```python
from build123d import *

# Parameters (mm, degrees)
F0_W     = 2
F0_H     = 0.5
F1_DEPTH = 13
F2_W     = 2
F2_H     = 6.25
F3_DEPTH = 11.37968


with BuildPart() as f1:
    # F0 (on Front) → F1 (new body)
    with BuildSketch(Plane.XZ):
        Polygon((-4.5, -3.75), (4.5, -3.75), (4.5, -3.25), (4.5, 3.75), (-4.5, 3.75), align=None)
        with Locations((5.5, -3.5)):
            Rectangle(F0_W, F0_H)
        Polygon((6.5, -3.25), (6.5, -3.75), (15.5, -3.75), (15.5, -3.25), (15.5, 3.75), (6.5, 3.75), align=None)
        with BuildLine():
            Line((-1.06066, 7.18934), (-4.5, 3.75))
            Line((-4.5, 3.75), (4.5, 3.75))
            Line((4.5, 3.75), (1.06066, 7.18934))
            ThreePointArc((1.06066, 7.18934), (0, 7.62868), (-1.06066, 7.18934))
        make_face()
        with Locations((16.5, -3.5)):
            Rectangle(F0_W, F0_H)
        with BuildLine():
            Line((9.93934, 7.18934), (6.5, 3.75))
            Line((6.5, 3.75), (15.5, 3.75))
            Line((15.5, 3.75), (12.06066, 7.18934))
            ThreePointArc((12.06066, 7.18934), (11, 7.62868), (9.93934, 7.18934))
        make_face()
        Polygon((17.5, -3.25), (17.5, -3.75), (26.5, -3.75), (26.5, -3.25), (26.5, 3.75), (17.5, 3.75), align=None)
        with Locations((27.5, -3.5)):
            Rectangle(F0_W, F0_H)
        with BuildLine():
            Line((20.93934, 7.18934), (17.5, 3.75))
            Line((17.5, 3.75), (26.5, 3.75))
            Line((26.5, 3.75), (23.06066, 7.18934))
            ThreePointArc((23.06066, 7.18934), (22, 7.62868), (20.93934, 7.18934))
        make_face()
        Polygon((28.5, -3.25), (28.5, -3.75), (37.5, -3.75), (37.5, -3.25), (37.5, 3.75), (28.5, 3.75), align=None)
        with Locations((38.5, -3.5)):
            Rectangle(F0_W, F0_H)
        with BuildLine():
            Line((31.93934, 7.18934), (28.5, 3.75))
            Line((28.5, 3.75), (37.5, 3.75))
            Line((37.5, 3.75), (34.06066, 7.18934))
            ThreePointArc((34.06066, 7.18934), (33, 7.62868), (31.93934, 7.18934))
        make_face()
        Polygon((39.5, -3.25), (39.5, -3.75), (48.5, -3.75), (48.5, -3.25), (48.5, 3.75), (39.5, 3.75), align=None)
        with Locations((49.5, -3.5)):
            Rectangle(F0_W, F0_H)
        with BuildLine():
            Line((42.93934, 7.18934), (39.5, 3.75))
            Line((39.5, 3.75), (48.5, 3.75))
            Line((48.5, 3.75), (45.06066, 7.18934))
            ThreePointArc((45.06066, 7.18934), (44, 7.62868), (42.93934, 7.18934))
        make_face()
    extrude(amount=-F1_DEPTH)

    # F2 (on face) → F3 (cut, through all)
    with BuildSketch(Plane(origin=(0, 0, -3.75), x_dir=(1, 0, 0), z_dir=(0, 0, -1))):
        with Locations((5.5, -3.125)):
            Rectangle(F2_W, F2_H)
        with Locations((5.5, -9.875)):
            Rectangle(F2_W, F2_H)
        with Locations((16.5, -3.125)):
            Rectangle(F2_W, F2_H)
        with Locations((16.5, -9.875)):
            Rectangle(F2_W, F2_H)
        with Locations((27.5, -3.125)):
            Rectangle(F2_W, F2_H)
        with Locations((27.5, -9.875)):
            Rectangle(F2_W, F2_H)
        with Locations((38.5, -3.125)):
            Rectangle(F2_W, F2_H)
        with Locations((38.5, -9.875)):
            Rectangle(F2_W, F2_H)
        with Locations((49.5, -3.125)):
            Rectangle(F2_W, F2_H)
        with Locations((49.5, -9.875)):
            Rectangle(F2_W, F2_H)
    extrude(amount=-F3_DEPTH, mode=Mode.SUBTRACT)


solid = f1.part
```
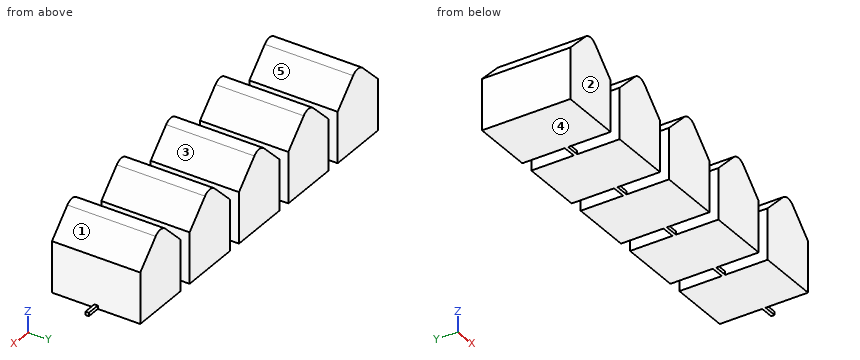
Here's how the part is built. I have some questions about the finished solid (model axes, mm). Face numbers are marked on the shaded views. A direction names the side the tool comes from. Coordinates: 2 decimals unless noted, no trailing zeros. Order: outer loops, then holes, each group sorted by start corner. A loop starts at its lowest first (then second) coordinate and runs counter-clockwise, first axis right, second up. Notation, with made-up numbers: M 45,58.25 L 66,58.25 A29 ccw 66,85.25 Z; hole C -25,16.5 d5. An arc over 180 degrees is marked long. Answer as a JSON object with one key per item and string values. Group by question number.
(1) I need wall thicknesses on probe 1 along X at (y, z) = (9.5, 3.75); probe 2 along X at (y, z) = (7.25, 5.25); probe 3 along Z at (x, y) = (2, 8.75). Which ranges of each line are inside material? Lowest first, please.
(2) Suppose I cut it at A-A, the plane y = 2. State how many separate pieces and enclosed holes the cut face has, then the cut area to 3 significant figures.
(3) Suppose I cut it at B-B, the plane z = 6. Please give me the cut outline in (x, y), then the cut area to 4 significant figures.
(4) Suppose I cut it at C-C, the plane z = -1.5. Please give me the cut outline in (x, y).
(5) Which directions (+Z, -Z, +X, -X, +Y, -Y) give clear straight access to the entire face, cutting with the end or side of a thin tool? Please do the marked faces 4 and 5.
(6) For pin 1 (3 mm diameter, centred on x = 27, y = 2.5, fed in from -Z); pin 2 (0.6 mm diameter, centred on x = 5.5, z = -3.5, fed in from -Y); pin 3 (2 mm diameter, centred on y = 3.5, z = -1.5, fed in from +X); pin 4 (2 mm diameter, centred on y = 9, z = 5.5, fed in from -X), each with a flat end and sliding along its axis, tell me the tip position at first contact or that it passes through.
(7) If we mould it in two halves opening along X, with no side actions, what happens to the marked faces 1, 2 and 3? For each: released by +X, released by -X, zero draft, split by the parting line, or undercut.
(8) Suppose I cut it at D-D, the plane x = 25. Please give me the cut outline in (y, z), then the cut area to 3 significant figures.
Values found:
{
 "1": {"probe 1": "x = -4.5 to 4.5, 6.5 to 15.5, 17.5 to 26.5, 28.5 to 37.5, 39.5 to 48.5", "probe 2": "x = -3 to 3, 8 to 14, 19 to 25, 30 to 36, 41 to 47", "probe 3": "z = -3.75 to 6.25"},
 "2": {"separate pieces": "5", "enclosed holes": "0", "area": "436 mm^2"},
 "3": {"outline": "M -2.25,0 L 2.25,0 L 2.25,13 L -2.25,13 Z; M 8.75,0 L 13.25,0 L 13.25,13 L 8.75,13 Z; M 19.75,0 L 24.25,0 L 24.25,13 L 19.75,13 Z; M 30.75,0 L 35.25,0 L 35.25,13 L 30.75,13 Z; M 41.75,0 L 46.25,0 L 46.25,13 L 41.75,13 Z", "area": "292.5 mm^2"},
 "4": {"outline": "M -4.5,0 L 4.5,0 L 4.5,13 L -4.5,13 Z; M 6.5,0 L 15.5,0 L 15.5,13 L 6.5,13 Z; M 17.5,0 L 26.5,0 L 26.5,13 L 17.5,13 Z; M 28.5,0 L 37.5,0 L 37.5,13 L 28.5,13 Z; M 39.5,0 L 48.5,0 L 48.5,13 L 39.5,13 Z"},
 "5": {"face 4": "-Z, +X, -X, +Y, -Y", "face 5": "+Z, +Y, -Y"},
 "6": {"pin 1": "stops at z = -3.75", "pin 2": "stops at y = 6.25", "pin 3": "stops at x = 48.5", "pin 4": "stops at x = -3.75"},
 "7": {"face 1": "released by +X", "face 2": "zero draft", "face 3": "undercut"},
 "8": {"outline": "M 0,-3.75 L 13,-3.75 L 13,5.25 L 0,5.25 Z", "area": "117 mm^2"}
}
